from build123d import *

# Parameters (mm, degrees)
F0_W     = 145
F0_H     = 80
F1_DEPTH = 2
F2_W     = 141
F2_H     = 76
F3_DEPTH = 1
F5_DEPTH = 25
F6_R     = 1
F7_DEPTH = 25


with BuildPart() as f1:
    # F0 (on Front) → F1 (new body)
    with BuildSketch(Plane.XZ):
        Rectangle(F0_W, F0_H)
    extrude(amount=F1_DEPTH)

    # F2 (on face) → F3 (join)
    with BuildSketch(Plane(origin=(0, 0, 0), x_dir=(-1, 0, 0), z_dir=(0, 1, 0))):
        Rectangle(F2_W, F2_H)
    extrude(amount=F3_DEPTH)

    # F4 (on face) → F5 (cut)
    with BuildSketch(Plane.XZ.offset(2)):
        with BuildLine():
            Line((3, -4.5), (3, 4.5))
            ThreePointArc((3, 4.5), (0, 7.5), (-3, 4.5))
            Line((-3, 4.5), (-3, -4.5))
            ThreePointArc((-3, -4.5), (0, -7.5), (3, -4.5))
        make_face()
    extrude(amount=-F5_DEPTH, mode=Mode.SUBTRACT)

    # F6 (on face) → F7 (cut)
    with BuildSketch(Plane.XZ.offset(2)):
        with Locations((-6.5, 16.5)):
            Circle(F6_R)
        with Locations((6.5, 16.5)):
            Circle(F6_R)
        with Locations((6.5, -7.5)):
            Circle(F6_R)
        with Locations((-6.5, -7.5)):
            Circle(F6_R)
        with Locations((-6.5, 4.5)):
            Circle(F6_R)
        with Locations((6.5, 4.5)):
            Circle(F6_R)
    extrude(amount=-F7_DEPTH, mode=Mode.SUBTRACT)


solid = f1.part
Input: part model. Units: mm. Frame: model coordinates. A direction names the side the tool comes from. Coordinates: 2 decimals unless noted, no trailing zeros. Loops run counter-clockwise (first coordinate to the right, second up) from the corner with the lowest first, then second, coordinate; pieces in that order, holes last. Notation, with made-up numbers: (33, -29.75) - (77, -29.75) arc R34 cw to (77, 6.25) - close; hole circle Ø8 at (52, 30). An arc over 180 degrees is marked (long way). Answer in a Markdown table with one row per item. Add a question column.
Item 1: Line query: line 1 along Z through (x, y) = (-6.5, -1); line 2 along X through (y, z) = (0.6, -7); line 3 along X through (y, z) = (0.75, -37). Output: solid intervals per line, ascending. Write a range as [from, to].
Item 2: Section query B-B on x = -45. Return the cut outline in (y, z).
Item 3: Contact query for a flat-ended pin moving along its axis: P1, Ø0.5, axis at x = 15, y = 0.5, coming from the +Z side. Output: stop coordinate, or through.
Item 4: Access query for faces 3 (the flat face through (-1, -2, 9)), 4 (the flat face through (-3, -1, 0)). Directions: +Z, -Z, +X, -X, +Y, -Y. A direction counts if a zero-diameter tool reaches every point of the face in a straight line with its end or side. Return the directions, or none.
Item 5: Mould query, pull axis Z, two halves, no side actions, for faces 1 (the flat face through (3, -1, 0)), 2 (the flat face through (1, 1, 9)). Classes: released by +Z, released by -Z, zero draft, split by the parting line, or undercut.
Item 6: Section query A-A on x = 0. Return the cut outline in (y, z).
Recorded:
| question | item | result |
|---|---|---|
| 1 | line 1 | [-40, -8.5], [-6.5, 3.5], [5.5, 15.5], [17.5, 40] |
| 1 | line 2 | [-70.5, -7.37], [-5.63, -1.66], [1.66, 5.63], [7.37, 70.5] |
| 1 | line 3 | [-70.5, 70.5] |
| 2 | outline | (-2, -40) - (0, -40) - (0, -38) - (1, -38) - (1, 38) - (0, 38) - (0, 40) - (-2, 40) - close |
| 3 | P1 | z = 38 |
| 4 | face 3 | +Z, -Z, +X, -X, -Y |
| 4 | face 4 | +Y, -Y |
| 5 | face 1 | undercut |
| 5 | face 2 | zero draft |
| 6 | outline | (-2, -40) - (0, -40) - (0, -38) - (1, -38) - (1, -7.5) - (-2, -7.5) - close; (-2, 7.5) - (1, 7.5) - (1, 38) - (0, 38) - (0, 40) - (-2, 40) - close |
